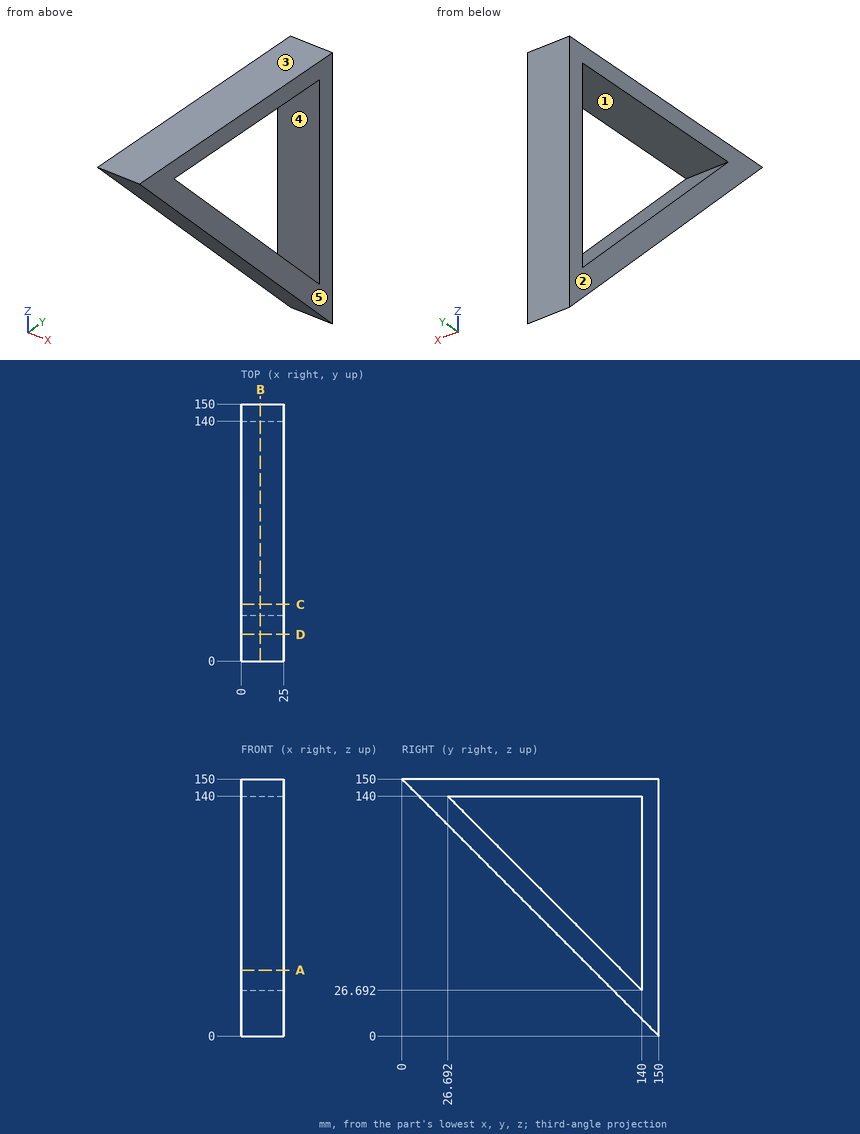
Can you work these out from the drawing? Everything is in mm from the part's minimum corner. A direction names the side the tool comes from. Round coordinates to 2 decimals unless told otherwise and drop trailing zeros. Loops run counter-clockwise (first coordinate to the right, second up) from the corner with the lowest first, then second, coordinate; pieces in that order, holes last. Notation, with made-up numbers: (-0.5, -18.75) -> (53.5, -18.75) arc R15 ccw to (53.5, 3.25) -> close; hole circle Ø8 at (19.5, 46.5). An arc over 180 degrees is marked (long way). Use CSV: the item, a comma, the result in double quotes.
(1) Suppose I cut it at A-A on z = 38.5. Write out the boundary of the cut face in (x, y), plus the area to 3 significant figures.
Return value:
outline,"(0, 111.5) -> (25, 111.5) -> (25, 128.19) -> (0, 128.19) -> close; (0, 140) -> (25, 140) -> (25, 150) -> (0, 150) -> close"
area,"667 mm²"
(2) Suppose I cut it at D-D on y = 15.5. Write out the boundary of the cut face in (x, z).
Return value:
outline,"(0, 134.5) -> (25, 134.5) -> (25, 150) -> (0, 150) -> close"
(3) If I drill on probe 1 along Y at (x, z) = (7.5, 31) (1 decimal); probe 2 along Y at (x, z) = (23.25, 87) (1 decimal); probe 3 along Z at (x, y) = (18.5, 68.5) (1 decimal), over which ranges is the centre line in solid material (lowest first)? Write a range as [from, to].
Return value:
probe 1,"y = [119, 135.7], [140, 150]"
probe 2,"y = [63, 79.7], [140, 150]"
probe 3,"z = [81.5, 98.2], [140, 150]"
(4) If we mould it in two halves opening along Z, with no side actions, what happens to the marked faces 1, 2 and 3? For each: +Z half, -Z half, draft (parallel to the pull), parting line (faces both ways), or undercut.
Return value:
face 1,"undercut"
face 2,"draft"
face 3,"+Z half"
(5) Suppose I cut it at C-C on y = 33. Write out the boundary of the cut face in (x, z).
Return value:
outline,"(0, 117) -> (25, 117) -> (25, 133.69) -> (0, 133.69) -> close; (0, 140) -> (25, 140) -> (25, 150) -> (0, 150) -> close"
(6) For the marked faces 4 and 5, which set-ups out of +Z, -Z, +X, -X, +Y, -Y let a thin tool reach every point of the face, with its end or its side?
Return value:
face 4,"+X, -X"
face 5,"+Z, -Z, +X, +Y, -Y"
(7) Suppose I cut it at B-B on x = 11.25. Write out the boundary of the cut face in (y, z).
Return value:
outline,"(0, 150) -> (150, 0) -> (150, 150) -> close; hole (26.69, 140) -> (140, 26.69) -> (140, 140) -> close"
(8) Will these pins go through, and if not, where does the flat tip stop? pin 1 Ø5 at (x, z) = (2.5, 50.5) entering from -Y; pin 2 Ø1.5 at (x, z) = (12, 119) entering from -Y; pin 3 Ø2 at (x, z) = (4, 122.5) entering from -Y.
Return value:
pin 1,"stops at y = 97"
pin 2,"stops at y = 30.25"
pin 3,"stops at y = 26.5"
